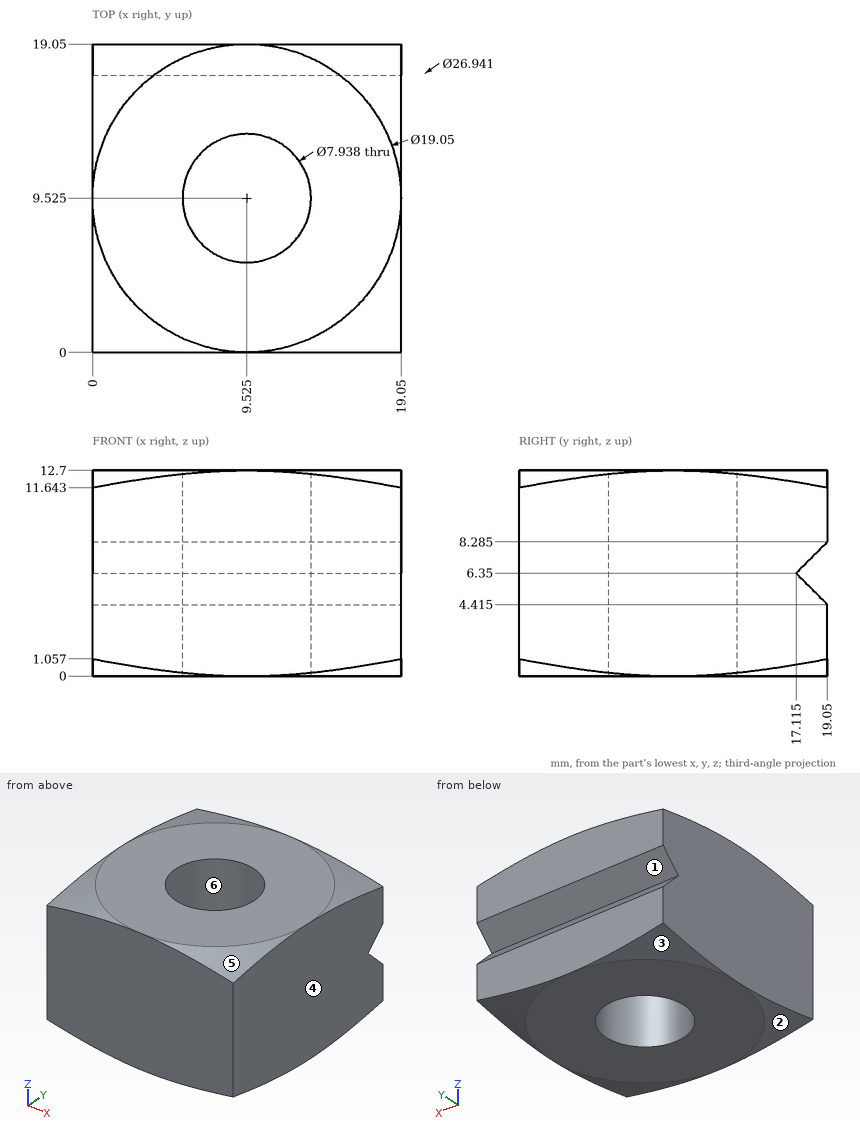
Study the drawing (mm; zero at the part's minimum x, y, z) and answer. A direction names the side the tool comes from. Round coordinates to 2 decimals unless told otherwise and drop trailing zeros.
1) A tool of negligible diameter and unlimited length cuts with its end or side. For the marked faces 1 and 2, from which of +Z, -Z, +X, -X, +Y, -Y can it reach the whole face along a straight path? Write none if from no direction.
2) Straight lines are drawn through the part: line 1 (Y direction, x = 7.5, z = 2.25); line 2 (Z direction, x = 3.5, y = 17.5) (1 decimal); line 3 (Y direction, x = 11.75, z = 6) (1 decimal). For each, find the intervals that lie inside material, in ascending order.
3) The mould has two halves that part along Y. Classify the marked faces 3, 4, 5 and 6: pulls with the +Y half, pulls with the -Y half, needs draft (parallel to the pull), parting line crosses it, or undercut.
Completed:
1. face 1: +X, -X, +Y
1. face 2: -Z, -X, -Y
2. line 1: y = 0 to 6.11, 12.94 to 19.05
2. line 2: z = 0.1 to 6, 6.7 to 12.6
2. line 3: y = 0 to 6.2, 12.8 to 17.5
3. face 3: pulls with the +Y half
3. face 4: needs draft
3. face 5: pulls with the -Y half
3. face 6: undercut
